from build123d import *

# Parameters (mm, degrees)
SKETCH_W      = 57
SKETCH_H      = 92
SKETCH_W_2    = 36.7
SKETCH_H_2    = 48.6
PAD_DEPTH     = 2
SKETCH001_R   = 2.25
SKETCH001_R_2 = 1.35
PAD001_DEPTH  = 6
SKETCH002_W   = 57
SKETCH002_H   = 92
SKETCH002_W_2 = 53
SKETCH002_H_2 = 88
PAD002_DEPTH  = 11
SKETCH007_W   = 38.7
SKETCH007_H   = 50.6
SKETCH007_W_2 = 36.7
SKETCH007_H_2 = 48.6
PAD005_DEPTH  = 2.4
SKETCH008_W   = 55
SKETCH008_H   = 90
SKETCH008_W_2 = 53
SKETCH008_H_2 = 88
PAD006_DEPTH  = 2
SKETCH009_R   = 2
POCKET_DEPTH  = 5


with BuildPart() as part:
    # Sketch → Pad (new body)
    with BuildSketch(Plane.XY):
        with Locations((21.690942, -23.151951)):
            Rectangle(SKETCH_W, SKETCH_H)
        with Locations((21.690942, -23.151951)):
            Rectangle(SKETCH_W_2, SKETCH_H_2, mode=Mode.SUBTRACT)
    extrude(amount=PAD_DEPTH)

    # Sketch001 (on Face10 of Pad) → Pad001 (join)
    with BuildSketch(Plane.XY.offset(2)):
        with Locations((4.340942, 5.348049)):
            Circle(SKETCH001_R)
        with Locations((4.340942, 5.348049)):
            Circle(SKETCH001_R_2, mode=Mode.SUBTRACT)
        with Locations((38.540942, 5.348049)):
            Circle(SKETCH001_R)
        with Locations((38.540942, 5.348049)):
            Circle(SKETCH001_R_2, mode=Mode.SUBTRACT)
        with Locations((4.340942, -56.151951)):
            Circle(SKETCH001_R)
        with Locations((4.340942, -56.151951)):
            Circle(SKETCH001_R_2, mode=Mode.SUBTRACT)
        with Locations((38.540942, -56.151951)):
            Circle(SKETCH001_R)
        with Locations((38.540942, -56.151951)):
            Circle(SKETCH001_R_2, mode=Mode.SUBTRACT)
    extrude(amount=PAD001_DEPTH)

    # Sketch002 (on Face5 of Pad001) → Pad002 (join)
    with BuildSketch(Plane.XY.offset(2)):
        with Locations((21.690942, -23.151951)):
            Rectangle(SKETCH002_W, SKETCH002_H)
        with Locations((21.690942, -23.151951)):
            Rectangle(SKETCH002_W_2, SKETCH002_H_2, mode=Mode.SUBTRACT)
    extrude(amount=PAD002_DEPTH)

    # Sketch007 (on Face15 of Pad002) → Pad005 (join)
    with BuildSketch(Plane.XY.offset(2)):
        with Locations((21.690942, -23.151951)):
            Rectangle(SKETCH007_W, SKETCH007_H)
        with Locations((21.690942, -23.151951)):
            Rectangle(SKETCH007_W_2, SKETCH007_H_2, mode=Mode.SUBTRACT)
    extrude(amount=PAD005_DEPTH)

    # Sketch008 (on Face13 of Pad002) → Pad006 (join)
    with BuildSketch(Plane.XY.offset(13)):
        with Locations((21.690942, -23.151951)):
            Rectangle(SKETCH008_W, SKETCH008_H)
        with Locations((21.690942, -23.151951)):
            Rectangle(SKETCH008_W_2, SKETCH008_H_2, mode=Mode.SUBTRACT)
    extrude(amount=PAD006_DEPTH)

    # Sketch009 (on Face5 of Pad006) → Pocket (cut)
    with BuildSketch(Plane(origin=(0, 22.848049, 0), x_dir=(-1, 0, 0), z_dir=(0, 1, 0))):
        with Locations((-38.190942, 10)):
            Circle(SKETCH009_R)
        with Locations((-33.190942, 10)):
            Circle(SKETCH009_R)
        with Locations((-28.190942, 10)):
            Circle(SKETCH009_R)
        with Locations((-23.190942, 10)):
            Circle(SKETCH009_R)
    extrude(amount=-POCKET_DEPTH, mode=Mode.SUBTRACT)


solid = part.part
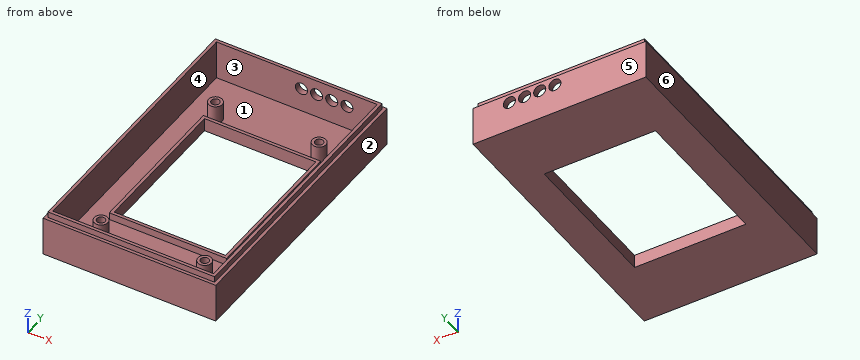
Here's how the part is built. I have some questions about the finished solid (model axes, mm). Face numbers are marked on the shaded views. A direction names the side the tool comes from. Round coordinates to 2 decimals unless told otherwise and drop trailing zeros. Loops run counter-clockwise (first coordinate to the right, second up) from the corner with the lowest first, then second, coordinate; pieces in that order, holes last. Notation, with made-up numbers: (22.25, 26.5) - (57.25, 26.5) arc R30 ccw to (57.25, 63.5) - close; hole circle Ø8 at (-39, 59.5). An arc over 180 degrees is marked (long way). One line per question, with ' | ' between items. Start each with the question number.
Q1. I want a section at D-D (x = 22.5). Write out the boundary of the cut face in (y, z), then the cut area to 3 significant figures.
Q2. I want a section at A-A (y = -16). Write out the boundary of the cut face in (x, z), then the cut area to 3 significant figures.
Q3. Will these pins go through, and if not, where does the flat tip stop? pin 1 (2 mm diameter, centred on x = 38, y = -56.5, fed in from +Z); pin 2 (2.5 mm diameter, centred on x = 4.34, y = 5.35, fed in from +Z); pin 3 (16 mm diameter, centred on x = 8.5, y = -38.5, fed in from +Z); pin 4 (4 mm diameter, centred on x = 38, y = -42, fed in from -Z).
Q4. I want a section at C-C (z = 10). Write out the boundary of the cut face in (x, y), then the cut area to 3 significant figures.
Q5. Please list where these lines run through material, in increasing order: line 1 (Y direction, x = 28.5, z = 4.25); line 2 (X direction, y = -56, z = 5); line 3 (X direction, y = -40, z = 3.25). Write a range as [from, to].
Q6. For the marked faces 1 and 2, which set-ups out of +Z, -Z, +X, -X, +Y, -Y let a thin tool reach every point of the face, with its end or its side?
Q7. We'd pull the mould along X, two halves only. Please class the marked faces 3, 4, 5 and 6: +X half, -X half, draft (parallel to the pull), parting line (faces both ways), or undercut.
Q8. I want a section at B-B (x = -3). Write out the boundary of the cut face in (y, z), then the cut area to 3 significant figures.
Response values:
1) outline: (-69.15, 0) - (-47.45, 0) - (-47.45, 4.4) - (-48.45, 4.4) - (-48.45, 2) - (-67.15, 2) - (-67.15, 15) - (-68.15, 15) - (-68.15, 13) - (-69.15, 13) - close; (1.15, 0) - (22.85, 0) - (22.85, 8.12) - (20.85, 8.12) - (20.85, 2) - (2.15, 2) - (2.15, 4.4) - (1.15, 4.4) - close; (20.85, 11.88) - (22.85, 11.88) - (22.85, 13) - (21.85, 13) - (21.85, 15) - (20.85, 15) - close | area: 132 mm²
2) outline: (-6.81, 0) - (3.34, 0) - (3.34, 4.4) - (2.34, 4.4) - (2.34, 2) - (-4.81, 2) - (-4.81, 15) - (-5.81, 15) - (-5.81, 13) - (-6.81, 13) - close; (40.04, 0) - (50.19, 0) - (50.19, 13) - (49.19, 13) - (49.19, 15) - (48.19, 15) - (48.19, 2) - (41.04, 2) - (41.04, 4.4) - (40.04, 4.4) - close | area: 93.4 mm²
3) pin 1: stops at z = 8 | pin 2: stops at z = 2 | pin 3: stops at z = 4.4 | pin 4: passes through
4) outline: (-6.81, -69.15) - (50.19, -69.15) - (50.19, 22.85) - (40.19, 22.85) - (40.19, 20.85) - (48.19, 20.85) - (48.19, -67.15) - (-4.81, -67.15) - (-4.81, 20.85) - (21.19, 20.85) - (21.19, 22.85) - (-6.81, 22.85) - close; (25.19, 20.85) - (26.19, 20.85) - (26.19, 22.85) - (25.19, 22.85) - close; (30.19, 20.85) - (31.19, 20.85) - (31.19, 22.85) - (30.19, 22.85) - close; (35.19, 20.85) - (36.19, 20.85) - (36.19, 22.85) - (35.19, 22.85) - close | area: 548 mm²
5) line 1: y = [-69.15, -67.15], [-48.45, -47.45], [1.15, 2.15], [20.85, 22.85] | line 2: x = [-6.81, -4.81], [2.1, 3], [5.68, 6.59], [36.3, 37.2], [39.88, 40.79], [48.19, 50.19] | line 3: x = [-6.81, -4.81], [2.34, 3.34], [40.04, 41.04], [48.19, 50.19]
6) face 1: +Z | face 2: +Z, -Z, +X, +Y, -Y
7) face 3: undercut | face 4: undercut | face 5: draft | face 6: -X half
8) outline: (-69.15, 0) - (22.85, 0) - (22.85, 13) - (21.85, 13) - (21.85, 15) - (20.85, 15) - (20.85, 2) - (-67.15, 2) - (-67.15, 15) - (-68.15, 15) - (-68.15, 13) - (-69.15, 13) - close | area: 232 mm²
